Drawing for the job (mm, zero at the part's lowest x, y, z). A direction names the side the tool comes from. Coordinates: 2 decimals unless noted, no trailing zeros. Write each loop counter-clockwise with the first axis right and the second up, starting at its lowest first coordinate (ties: lowest second). Pieces come first, ordered by that corner, then holes.
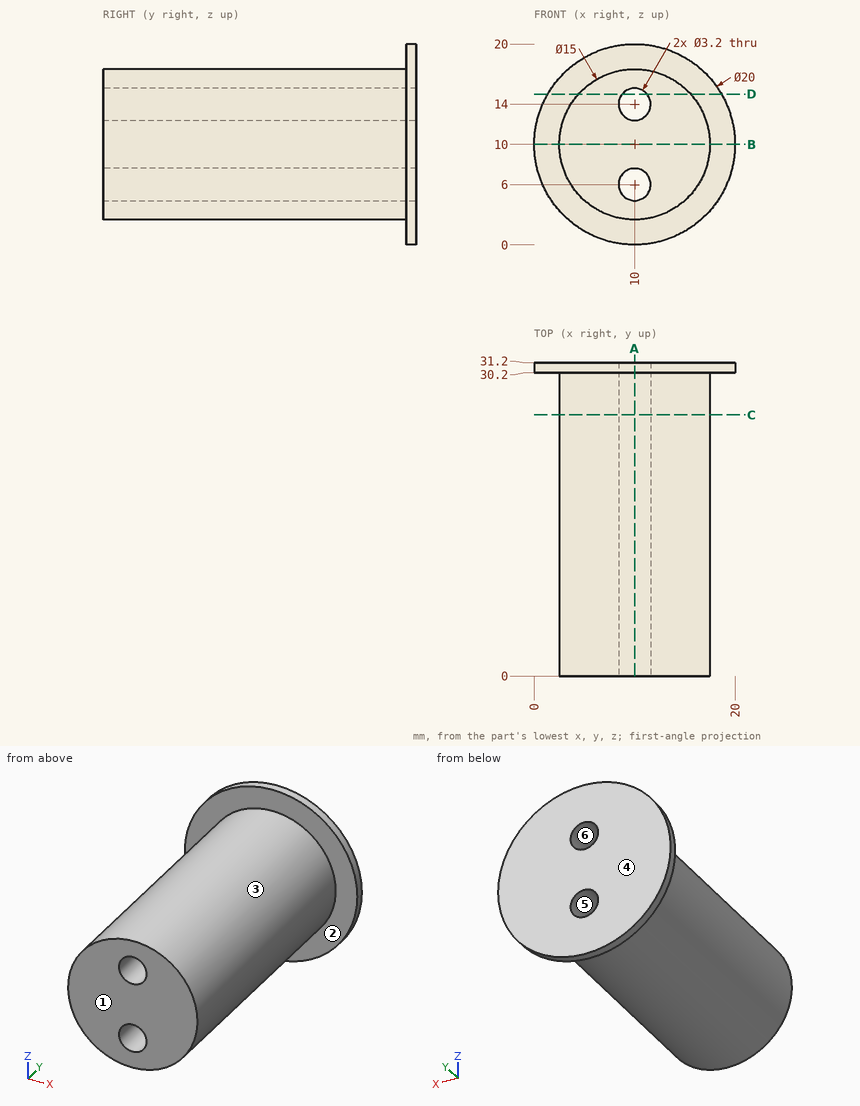
Item 1: Which spindle directions (+Z, -Z, +X, -X, +Y, -Y) get a long thin tool onto all of the face, cutting with end or side? Do the marked faces 1 and 2. Say none if no direction does.
Item 2: Saw through at D-D, the plane z = 15. Write the cut outline in (x, y), and give its area (3 significant figures).
Item 3: Saw through at C-C, the plane y = 26. Write the cut outline in (x, z), and give its area (3 significant figures).
Item 4: Flat gauge pins, fed straight in: pin 1 Ø5 at (y, z) = (7, 4.5) entering from +X; pin 2 Ø2.5 at (x, z) = (10, 6) entering from -Y; pin 3 Ø6 at (x, y) = (14.5, 10.5) entering from +Z; pin 4 Ø5 at (y, z) = (3.5, 16) entering from +X. Where does each tip first touch, or does it go through?
Item 5: Saw through at B-B, the plane z = 10. Write the cut outline in (x, y), and give its area (3 significant figures).
Item 6: Saw through at A-A, the plane x = 10. Write the cut outline in (y, z), and give its area (3 significant figures).
Item 7: Wall check: line 1 along Y through (x, z) = (16.25, 4.75); line 2 along X through (y, z) = (2.5, 6); line 3 along Z through (x, y) = (10.5, 24). Give the ranges that are in metal, low to high.
Item 8: Two-plate mould, pull along X, no slides. Class the marked faces 3, 4, 5 and 6: +X half, -X half, draft (parallel to the pull), parting line (faces both ways), or undercut.
Working result:
1. face 1: +Z, -Z, +X, -X, -Y
1. face 2: -Y
2. outline: (1.34, 30.2) - (4.41, 30.2) - (4.41, 0) - (8.75, 0) - (8.75, 31.2) - (1.34, 31.2) - close; (11.25, 0) - (15.59, 0) - (15.59, 30.2) - (18.66, 30.2) - (18.66, 31.2) - (11.25, 31.2) - close
2. area: 277 mm2
3. outline: circle Ø15 at (10, 10); hole circle Ø3.2 at (10, 6); hole circle Ø3.2 at (10, 14)
3. area: 161 mm2
4. pin 1: stops at x = 16.87
4. pin 2: passes through
4. pin 3: stops at z = 17.35
4. pin 4: stops at x = 16.63
5. outline: (0, 30.2) - (2.5, 30.2) - (2.5, 0) - (17.5, 0) - (17.5, 30.2) - (20, 30.2) - (20, 31.2) - (0, 31.2) - close
5. area: 473 mm2
6. outline: (0, 2.5) - (30.2, 2.5) - (30.2, 0) - (31.2, 0) - (31.2, 4.4) - (0, 4.4) - close; (0, 7.6) - (31.2, 7.6) - (31.2, 12.4) - (0, 12.4) - close; (0, 15.6) - (31.2, 15.6) - (31.2, 20) - (30.2, 20) - (30.2, 17.5) - (0, 17.5) - close
6. area: 273 mm2
7. line 1: y = 30.2 to 31.2
7. line 2: x = 3.66 to 8.4, 11.6 to 16.34
7. line 3: z = 2.52 to 4.48, 7.52 to 12.48, 15.52 to 17.48
8. face 3: parting line
8. face 4: draft
8. face 5: undercut
8. face 6: undercut
